The figure shows three views and two pictorial views of one solid part (mm, origin at its lowest corner). Answer the questions. A direction names the side the tool comes from. Coordinates: 2 decimals unless noted, no trailing zeros. Order: outer loops, then holes, each group sorted by start corner. A loop starts at its lowest first (then second) coordinate and runs counter-clockwise, first axis right, second up. Notation, with made-up numbers: M 69,46.25 L 101,46.25 A21 cw 101,78.25 Z; hole C -28.5,32.5 d7. An arc over 180 degrees is marked long. Use a Markdown table: item, result.
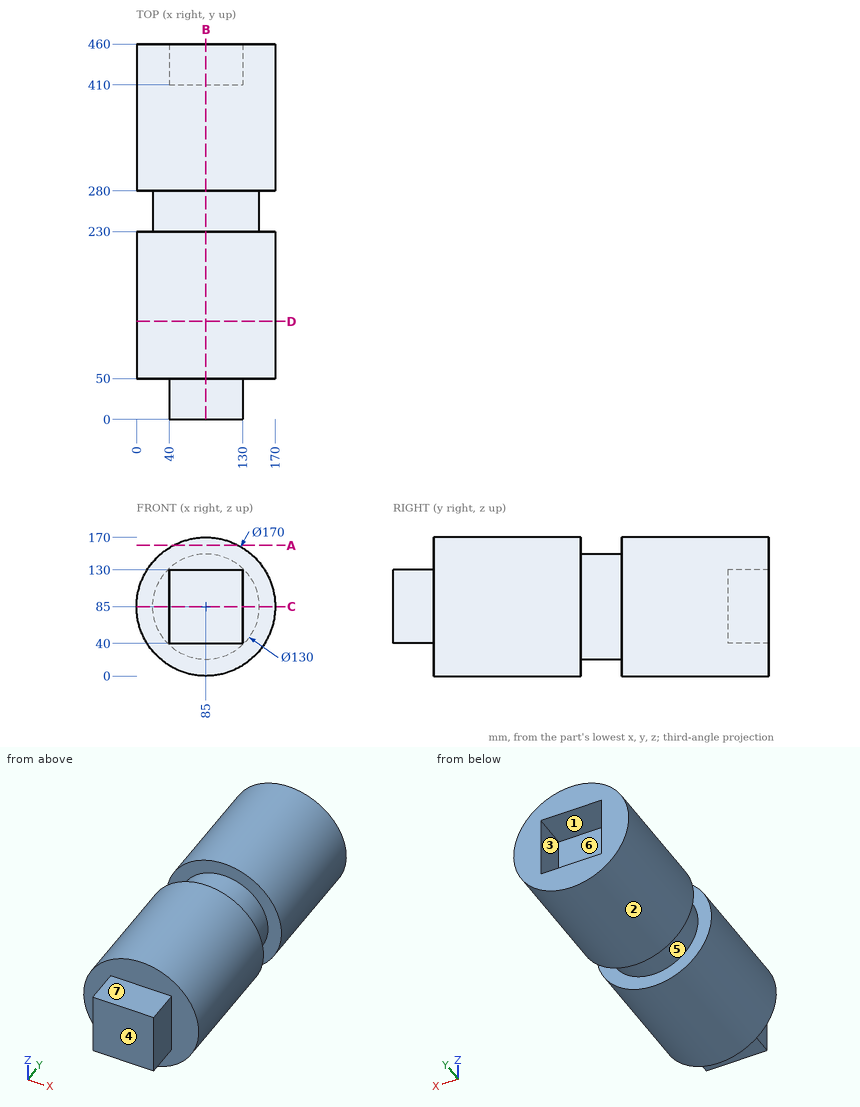
1. Section B-B on x = 85 is taken. Determine the outline of the cut face in (y, z), then the cut area to 3 significant figures.
Answers below:
| item | result |
|---|---|
| outline | M 0,40 L 50,40 L 50,0 L 230,0 L 230,20 L 280,20 L 280,0 L 460,0 L 460,40 L 410,40 L 410,130 L 460,130 L 460,170 L 280,170 L 280,150 L 230,150 L 230,170 L 50,170 L 50,130 L 0,130 Z |
| area | 67,700 mm² |
2. Find the intervals of material crossed by probe 1 along Y at (x, z) = (79.5, 82); probe 2 along Y at (x, z) = (137.5, 48); probe 3 along Z at (x, y) = (82.5, 241.5), in increasing order.
Answers below:
| item | result |
|---|---|
| probe 1 | 0 to 410 |
| probe 2 | 50 to 460 |
| probe 3 | 20.05 to 149.95 |
3. Section C-C on z = 85 is taken. Determine the outline of the cut face in (x, y), then the cut area to 3 significant figures.
Answers below:
| item | result |
|---|---|
| outline | M 0,50 L 40,50 L 40,0 L 130,0 L 130,50 L 170,50 L 170,230 L 150,230 L 150,280 L 170,280 L 170,460 L 130,460 L 130,410 L 40,410 L 40,460 L 0,460 L 0,280 L 20,280 L 20,230 L 0,230 Z |
| area | 67,700 mm² |
4. Section A-A on z = 160 is taken. Determine the outline of the cut face in (x, y).
Answers below:
| item | result |
|---|---|
| outline | M 45,50 L 125,50 L 125,230 L 45,230 Z; M 45,280 L 125,280 L 125,460 L 45,460 Z |
5. Flat-ended cylindrical pins translate along their axes: P1, Ø5, axis at x = 76.5, y = 267, coming from the -Z side; P2, Ø2, axis at x = 110, z = 36.5, coming from the -Y side; P3, Ø25, axis at x = 71, y = 35, coming from the -Z side. Find the tip coordinate at first contact, or state that the pin passes through.
Answers below:
| item | result |
|---|---|
| P1 | z = 20.28 |
| P2 | y = 50 |
| P3 | z = 40 |
6. For a pull along Z with two mould halves and no side action, classify the marked faces 1, 2, 3 and 4 as +Z half, -Z half, draft (parallel to the pull), parting line (faces both ways), or undercut.
Answers below:
| item | result |
|---|---|
| face 1 | undercut |
| face 2 | parting line |
| face 3 | undercut |
| face 4 | draft |
7. Section D-D on y = 120 is taken. Determine the outline of the cut face in (x, z), then the cut area to 3 significant figures.
Answers below:
| item | result |
|---|---|
| outline | C 85,85 d170 |
| area | 22,700 mm² |
8. For the marked faces 5, 6 and 7, determine the directions among +Z, -Z, +X, -X, +Y, -Y from which every point of the face is accessible in a straight line to the end or side of a thin tool.
Answers below:
| item | result |
|---|---|
| face 5 | none |
| face 6 | +Y |
| face 7 | +Z, +X, -X, -Y |
